CAD build for the part. Positions are in the model's coordinates, mm. Give positions to 0.01 mm unless a question says otherwise; leave off trailing zeros. Order: outer loops, then holes, each group sorted by start corner. A loop starts at its lowest first (then second) coordinate and runs counter-clockwise, first axis right, second up.
Item 1: Band-saw the part on C-C on x = 5.5. Give the cut face in (y, z), plus the area to 3 significant figures.
Item 2: Flat gauge pins, fed straight in: P1, Ø1, axis at y = 2, z = -10.5, coming from the -X side; P2, Ø10, axis at x = 28, z = -14.5, coming from the +Y side; P3, Ø2, axis at x = 27.257, z = -9.25, coming from the -Y side. Where does each tip first touch, or does it go through?
Item 3: Band-saw the part on A-A on y = 3. Give the cut face in (x, z).
Item 4: Band-saw the part on B-B on z = -3.5. Give the cut face in (x, y), plus the area to 3 significant figures.
Item 5: Wall check: L1, parallel to X at y = 2.2, z = -9.25; L2, parallel to X at y = 3.4, z = -9.25; L3, parallel to X at y = 5.5, z = -16.75. Give the ranges that are in metal, low to high.
Autodesk Inventor part; units mm, degrees
ref_plane "YZ Plane" through (0, 0, 0) normal (1, 0, 0) x (0, 1, 0)
ref_plane "XZ Plane" through (0, 0, 0) normal (0, 1, 0) x (-1, 0, 0)
ref_plane "XY Plane" through (0, 0, 0) normal (0, 0, 1) x (1, 0, 0)
sketch "Szkic1" plane through (0, 0, 0) normal (1, 0, 0) x (0, 1, 0)
  line L0 (0, 0) -> (20, 0)
  line L1 (20, 0) -> (20, -24.25)
  line L2 (20, -24.25) -> (0, -24.25)
  line L3 (0, -24.25) -> (0, 0)
  line L4 (0, 0) -> (20, -20)
  dimension "d0" = 20
  dimension "d1" = 24.25
  dimension "d4" = 45
extrude "Wyciągnięcie proste1" add sketch "Szkic1" along normal blind 32.257 contours L4 L1 L2 L3
sketch "Szkic2" plane through (0, 0, -24.25) normal (0, 0, -1) x (-1, 0, 0)
  line L0 (0, 0) -> (0, 20)
  line L1 (0, 0) -> (0, 20)
  line L2 (0, 0) -> (-20, 20)
  line L3 (0, 20) -> (-32.257, 20)
  dimension "d5" = 45
extrude "Wyciągnięcie proste2" cut sketch "Szkic2" against normal up to next
sketch "Szkic3" plane through (32.257, 0, -24.25) normal (0, -1, 0) x (1, 0, 0)
  line L0 (0, 24.25) -> (0, 0)
  line L1 (-32.257, 24.25) -> (0, 24.25)
  line L2 (-32.257, 24.25) -> (-32.257, 0)
  line L3 (-32.257, 0) -> (0, 0)
  point P0 (-5, 15)
  point P1 (-24.5, 7)
  dimension "d8" = 5
  dimension "d38" = 24.5
  dimension "d39" = 7
  dimension "d40" = 15
hole "Otwór1" at (27.257, 0, -9.25) at (7.757, 0, -17.25) direction (0, 1, 0) diameter 2.459 depth 5 tip angle 118
sketch "Szkic4" plane through (0, 0, 0) normal (0, 0.7071, 0.7071) x (1, 0, 0)
  line L0 (20, 28.2843) -> (32.257, 28.2843)
  line L1 (32.257, 28.2843) -> (32.257, 0)
  point P0 (0, 0)
  point P1 (25.9815, 18.6912)
  dimension "d19" = 9.5931
  dimension "d20" = 6.2755
hole "Otwór2" at (25.9815, 13.2167, -13.2167) direction (0, -0.7071, -0.7071) diameter 2.459 depth 5 tip angle 118
sketch "Szkic5" plane through (0, 0, -24.25) normal (-0.7071, 0.7071, 0) x (-0.7071, -0.7071, 0)
  line L0 (0, 24.25) -> (0, 0)
  line L1 (0, 0) -> (-28.2843, 0)
  line L2 (-28.2843, 0) -> (-28.2843, 4.25)
  point P0 (-11.9843, 6)
  dimension "d29" = 6
  dimension "d37" = 16.3
hole "Otwór3" at (8.4742, 8.4742, -18.25) direction (0.7071, -0.7071, 0) diameter 2.459 depth 5 tip angle 118
properties part number "MocowanieBok2"
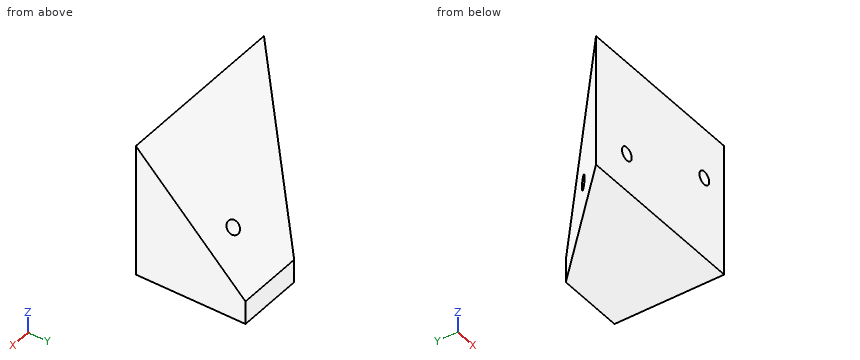
The answers:
1. outline: (0, -24.25) - (5.5, -24.25) - (5.5, -5.5) - (0, 0) - close
1. area: 118 mm2
2. P1: stops at x = 1.5
2. P2: stops at y = 19.5
2. P3: stops at y = 5.14
3. outline: (3, -24.25) - (32.26, -24.25) - (32.26, -3) - (3, -3) - close; hole circle Ø2.46 at (7.76, -17.25); hole circle Ø2.46 at (27.26, -9.25)
4. outline: (0, 0) - (32.26, 0) - (32.26, 3.5) - (3.5, 3.5) - close
4. area: 107 mm2
5. L1: x = 2.2 to 26.03, 28.49 to 32.26
5. L2: x = 3.4 to 26.03, 28.49 to 32.26
5. L3: x = 5.5 to 32.26
